from build123d import *

# Parameters (mm, degrees)
BOSS_EXTRUDE1_DEPTH = 12


with BuildPart() as part:
    # Sketch1 → Boss-Extrude1 (new body)
    with BuildSketch(Plane(origin=(0, 0, 0), x_dir=(0, 0, -1), z_dir=(1, 0, 0))):
        with BuildLine():
            Line((73, 94), (25, 94))
            Line((25, 94), (25, 65.097722286))
            ThreePointArc((25, 65.097722286), (25.604754635, 62.714065813), (27.272727273, 60.90702026))
            ThreePointArc((27.272727273, 60.90702026), (0, -31), (-27.272727273, 60.90702026))
            ThreePointArc((-27.272727273, 60.90702026), (-25.604754635, 62.714065813), (-25, 65.097722286))
            Line((-25, 65.097722286), (-25, 94))
            Line((-25, 94), (-73, 94))
            Line((-73, 94), (-73, -94))
            Line((-73, -94), (73, -94))
            Line((73, -94), (73, 94))
        make_face()
    extrude(amount=BOSS_EXTRUDE1_DEPTH)


solid = part.part
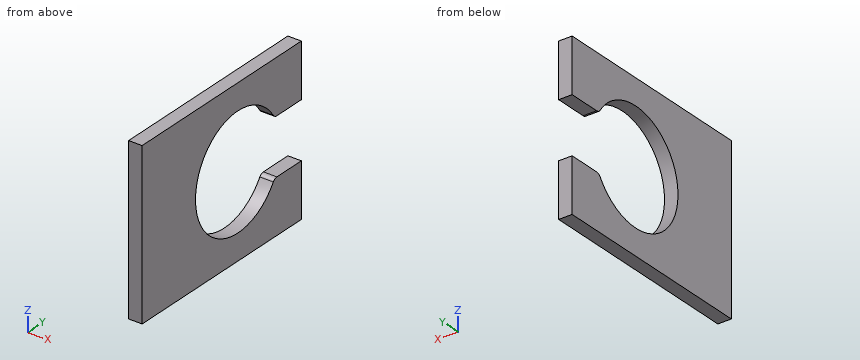
Geometry: final body of the model. Coordinates: model frame, mm. Coordinates: 2 decimals unless noted, no trailing zeros. Loops run counter-clockwise (first coordinate to the right, second up) from the corner with the lowest first, then second, coordinate; pieces in that order, holes last. Notation, with made-up numbers: M -7.75,10 L 46.25,10 A14 cw 46.25,27 Z; hole C 30.25,32 d9. An arc over 180 degrees is marked long. One line per item, written item: value. Start each with the question number.
1) Cut plane B-B (z = -30). Return loops of the section in (x, y), then the cut area to 3 significant figures.
2) Cut plane C-C (x = 3.5). Return loops of the section in (y, z).
3) Pin query (flat end, axial travel): P1, Ø4, axis at y = -44.5, z = -45, coming from the -X side; P2, Ø6, axis at x = 6, z = 17.5, coming from the +Y side; P3, Ø6, axis at x = 2, z = -20.5, coming from the +Y side. Return the tip coordinate at first contact, or that it passes through.
4) Material intervals for L1, parallel to Z at x = 9, y = 19; L2, parallel to Z at x = 8.5, y = 84; L3, parallel to Y at x = 7.75, z = 0, sorted ascending. Write a range as from..to.
5) Cut plane D-D (z = 1). Return loops of the section in (x, y), then the cut area to 3 significant figures.
6) Cut plane A-A (y = 19). Return loops of the section in (x, z).
Evaluation:
1. outline: M 0,-94 L 12,-94 L 12,-21 L 0,-21 Z; M 0,59 L 12,59 L 12,94 L 0,94 Z
1. area: 1,300 mm^2
2. outline: M -94,-73 L 94,-73 L 94,-25 L 65.1,-25 A5 ccw 60.91,-27.27 A50 cw long 60.91,27.27 A5 ccw 65.1,25 L 94,25 L 94,73 L -94,73 Z
3. P1: x = 0
3. P2: y = -26.6
3. P3: y = -25.13
4. L1: -73..-50, 50..73
4. L2: -73..-25, 25..73
4. L3: -94..-31
5. outline: M 0,-94 L 12,-94 L 12,-30.99 L 0,-30.99 Z
5. area: 756 mm^2
6. outline: M 0,-73 L 12,-73 L 12,-50 L 0,-50 Z; M 0,50 L 12,50 L 12,73 L 0,73 Z
